Verification items for the finished model (mm, model axes). Face numbers are marked on the shaded views. A direction names the side the tool comes from. Round coordinates to 2 decimals unless told otherwise and drop trailing zeros. Write each loop counter-clockwise with the first axis right and the second up, starting at its lowest first coordinate (ties: lowest second). Pieces come first, ordered by that corner, then holes.
from build123d import *

# Parameters (mm, degrees)
SKETCH2_R           = 15
SKETCH2_R_2         = 5
BOSS_EXTRUDE1_DEPTH = 1
BOSS_EXTRUDE2_START = 1
SKETCH2_3_R         = 5
BOSS_EXTRUDE2_DEPTH = 4
BOSS_EXTRUDE3_START = 5
SKETCH2_5_R         = 15
SKETCH2_5_R_2       = 5
BOSS_EXTRUDE3_DEPTH = 1
BOSS_EXTRUDE4_START = 6
SKETCH2_6_R         = 5
BOSS_EXTRUDE4_DEPTH = 4
BOSS_EXTRUDE5_START = 10
SKETCH2_7_R         = 15
SKETCH2_7_R_2       = 5
BOSS_EXTRUDE5_DEPTH = 1
SKETCH3_R           = 2.375
CUT_EXTRUDE1_DEPTH  = 2
CUT_EXTRUDE6_START  = -3
SKETCH3_4_R         = 2.8
CUT_EXTRUDE6_DEPTH  = 8
SKETCH3_5_R         = 0.6
CUT_EXTRUDE7_DEPTH  = 3


with BuildPart() as part:
    # Sketch2 → Boss-Extrude1 (new body)
    with BuildSketch(Plane(origin=(0, 0, 0), x_dir=(0, 0, -1), z_dir=(1, 0, 0))):
        Circle(SKETCH2_R)
        Circle(SKETCH2_R_2, mode=Mode.SUBTRACT)
        Circle(SKETCH2_R_2)
    extrude(amount=BOSS_EXTRUDE1_DEPTH)

    # Sketch2<3> → Boss-Extrude2 (add)
    with BuildSketch(Plane(origin=(0, 0, 0), x_dir=(0, 0, -1), z_dir=(1, 0, 0)).offset(BOSS_EXTRUDE2_START)):
        Circle(SKETCH2_3_R)
    extrude(amount=BOSS_EXTRUDE2_DEPTH)

    # Sketch2<5> → Boss-Extrude3 (add)
    with BuildSketch(Plane(origin=(0, 0, 0), x_dir=(0, 0, -1), z_dir=(1, 0, 0)).offset(BOSS_EXTRUDE3_START)):
        Circle(SKETCH2_5_R)
        Circle(SKETCH2_5_R_2, mode=Mode.SUBTRACT)
        Circle(SKETCH2_5_R_2)
    extrude(amount=BOSS_EXTRUDE3_DEPTH)

    # Sketch2<6> → Boss-Extrude4 (add)
    with BuildSketch(Plane(origin=(0, 0, 0), x_dir=(0, 0, -1), z_dir=(1, 0, 0)).offset(BOSS_EXTRUDE4_START)):
        Circle(SKETCH2_6_R)
    extrude(amount=BOSS_EXTRUDE4_DEPTH)

    # Sketch2<7> → Boss-Extrude5 (add)
    with BuildSketch(Plane(origin=(0, 0, 0), x_dir=(0, 0, -1), z_dir=(1, 0, 0)).offset(BOSS_EXTRUDE5_START)):
        Circle(SKETCH2_7_R)
        Circle(SKETCH2_7_R_2, mode=Mode.SUBTRACT)
        Circle(SKETCH2_7_R_2)
    extrude(amount=BOSS_EXTRUDE5_DEPTH)

    # Sketch3 → Cut-Extrude1 (cut)
    with BuildSketch(Plane.ZY):
        Circle(SKETCH3_R)
    extrude(amount=-CUT_EXTRUDE1_DEPTH, mode=Mode.SUBTRACT)

    # Sketch3<4> → Cut-Extrude6 (cut)
    with BuildSketch(Plane.ZY.offset(CUT_EXTRUDE6_START)):
        Circle(SKETCH3_4_R)
    extrude(amount=-CUT_EXTRUDE6_DEPTH, mode=Mode.SUBTRACT)

    # Sketch3<5> → Cut-Extrude7 (cut)
    with BuildSketch(Plane.ZY):
        Circle(SKETCH3_5_R)
    extrude(amount=-CUT_EXTRUDE7_DEPTH, mode=Mode.SUBTRACT)


solid = part.part
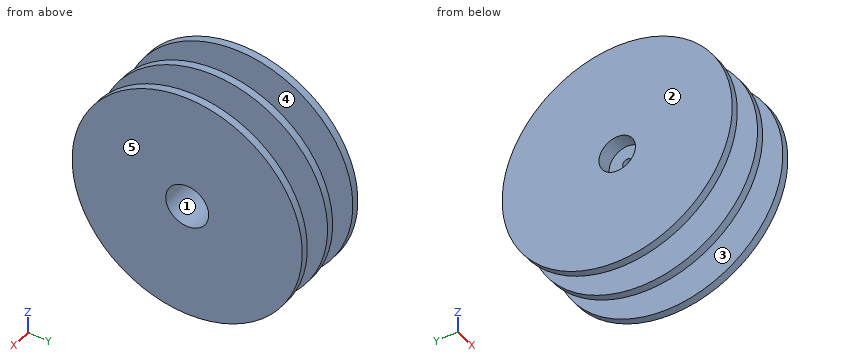
Q1. Material ranges on line 1 along X through (y, z) = (-4.75, -5.75); line 2 along Y through (x, z) = (2.5, -0.25); line 3 along Z through (x, y) = (4.5, -1), recorded low to high.
Recorded:
line 1: x = 0 to 1, 5 to 6, 10 to 11
line 2: y = -4.99 to -0.55, 0.55 to 4.99
line 3: z = -4.9 to -2.62, 2.62 to 4.9
Q2. Tool access check on the marked faces 4 and 5. Record the directions out of +Z, -Z, +X, -X, +Y, -Y that give a thin tool (end or side, any length) a straight path to the whole face; none if there is none.
Recorded:
face 4: none
face 5: +Z, -Z, +X, +Y, -Y
Q3. Sectioned sample at D-D (x = 10.5). Enter the section's corners in (y, z).
Recorded:
outline: circle Ø30 at (0, 0); hole circle Ø5.6 at (0, 0)
Q4. Depth check by flat-ended pin: P1, Ø1.6, axis at y = 0, z = 0, coming from the -X side; P2, Ø1.7, axis at y = 0, z = 0.5, coming from the +X side; P3, Ø3, axis at x = 3, y = 7, coming from the -Z side. Enter the tip coordinate at first touch or a pass-through.
Recorded:
P1: stops at x = 2
P2: stops at x = 3
P3: passes through
Q5. Sectioned sample at C-C (x = 8.25). Enter the section's corners in (y, z), plus the area to 3 significant figures.
Recorded:
outline: circle Ø10 at (0, 0); hole circle Ø5.6 at (0, 0)
area: 53.9 mm2
Q6. Release check for a two-part mould opening along X. For the marked faces 1, 2 and 3 record: released by +X, released by -X, zero draft, split by the parting line, or undercut.
Recorded:
face 1: zero draft
face 2: released by -X
face 3: undercut
